The listing builds one solid part. Answer for the finished solid, in the listing's coordinates (mm). Face numbers are marked on the shaded views. A direction names the side the tool comes from. Coordinates: 2 decimals unless noted, no trailing zeros. Loops run counter-clockwise (first coordinate to the right, second up) from the corner with the lowest first, then second, coordinate; pieces in that order, holes last. Notation, with made-up numbers: (88.5, 2) - (110.5, 2) arc R12 cw to (110.5, 10) - close; hole circle Ø8 at (56.25, 55.25). An arc over 180 degrees is marked (long way). Return JSON: item names as keys, results as strings. Group by question number.
1. The mould has two halves that part along Y. Classify the marked faces 1, 2 and 3: pulls with the +Y half, pulls with the -Y half, needs draft (parallel to the pull), parting line crosses it, or undercut.
2. Which of the six approach directions +Z, -Z, +X, -X, +Y, -Y give full straight-line access (tool end or side, diameter ignored) to the marked faces 4, 5 and 6?
3. Section A-A (x = 0) is taken. Write down the section's boundary in (y, z) (3 decimals), and give its area (3 significant figures).
4. Each of these flat-tipped pins is pushed along its axis until it touches: P1, Ø11, axis at x = 2, z = 18, coming from the -Y side (3 decimals); P2, Ø4, axis at x = 3.5, y = -15.5, coming from the +Z side. Where does it stop, or does it pass through?
5. Find the intervals of material crossed by line 1 along Y through (x, z) = (0, 2) (3 decimals); line 2 along Y through (x, z) = (-5, 4) (3 decimals); line 3 along Y through (x, z) = (8.5, 15.75) (3 decimals), in increasing order.
6. Section B-B (y = -16.25) is taken. Write down the section's boundary in (x, z) (3 decimals).
7. Section C-C (z = 6) is taken. Write down the section's boundary in (x, y) (3 decimals).
8. Section D-D (y = -3) is taken. Write down the section's boundary in (x, z) (3 decimals), and give its area (3 significant figures).
```python
from build123d import *

# Parameters (mm, degrees)
F0_W      = 21.85
F0_H      = 15.85
F1_DEPTH  = 25
F3_DEPTH  = 22
F4_R      = 2.4
F5_DEPTH  = 3.001
F6_W      = 21.85
F6_H      = 14
F6_R      = 2.4
F7_DEPTH  = 3
F9_DEPTH  = 2
F11_DEPTH = 2


with BuildPart() as f1:
    # F0 (on Top) → F1 (new body)
    with BuildSketch(Plane.XY):
        Rectangle(F0_W, F0_H)
    extrude(amount=F1_DEPTH)

    # F2 (on face) → F3 (cut, through all)
    with BuildSketch(Plane.XY.offset(25)):
        with BuildLine():
            Line((3.2894660941, 3.825), (-3.2894660941, 3.825))
            ThreePointArc((-3.2894660941, 3.825), (-6.825, 3.825), (-6.825, 0.2894660941))
            Line((-6.825, 0.2894660941), (-6.825, -0.2894660941))
            ThreePointArc((-6.825, -0.2894660941), (-6.825, -3.825), (-3.2894660941, -3.825))
            Line((-3.2894660941, -3.825), (3.2894660941, -3.825))
            ThreePointArc((3.2894660941, -3.825), (6.825, -3.825), (6.825, -0.2894660941))
            Line((6.825, -0.2894660941), (6.825, 0.2894660941))
            ThreePointArc((6.825, 0.2894660941), (6.825, 3.825), (3.2894660941, 3.825))
        make_face()
    extrude(amount=-F3_DEPTH, mode=Mode.SUBTRACT)

    # F4 (on face) → F5 (cut, through all)
    with BuildSketch(Plane.XY.offset(3)):
        Circle(F4_R)
    extrude(amount=-F5_DEPTH, mode=Mode.SUBTRACT)

    # F6 (on Top) → F7 (join)
    with BuildSketch(Plane.XY):
        with Locations((0, -14.925)):
            Rectangle(F6_W, F6_H)
        with Locations((0, -14.925)):
            Circle(F6_R, mode=Mode.SUBTRACT)
    extrude(amount=F7_DEPTH)

    # F8 (on face) → F9 (join)
    with BuildSketch(Plane(origin=(-10.925, 0, 0), x_dir=(0, -1, 0), z_dir=(-1, 0, 0))):
        Polygon((21.925, 3), (7.925, 17), (7.925, 3), align=None)
    extrude(amount=-F9_DEPTH)

    # F10 (on face) → F11 (join)
    with BuildSketch(Plane.YZ.offset(10.925)):
        Polygon((-7.925, 3), (-7.925, 17), (-21.925, 3), align=None)
    extrude(amount=-F11_DEPTH)


solid = f1.part
```
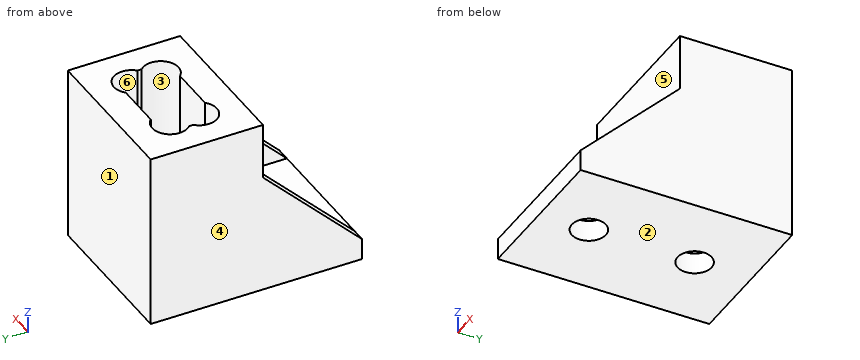
The answers:
{
 "1": {"face 1": "pulls with the +Y half", "face 2": "needs draft", "face 3": "undercut"},
 "2": {"face 4": "+Z, -Z, -X, +Y, -Y", "face 5": "+Z, -Y", "face 6": "+Z"},
 "3": {"outline": "(-21.925, 0) - (-17.325, 0) - (-17.325, 3) - (-21.925, 3) - close; (-12.525, 0) - (-2.4, 0) - (-2.4, 3) - (-3.825, 3) - (-3.825, 25) - (-7.925, 25) - (-7.925, 3) - (-12.525, 3) - close; (2.4, 0) - (7.925, 0) - (7.925, 25) - (3.825, 25) - (3.825, 3) - (2.4, 3) - close", "area": "241 mm2"},
 "4": {"P1": "stops at y = -7.925", "P2": "stops at z = 3"},
 "5": {"line 1": "y = -21.925 to -17.325, -12.525 to -2.4, 2.4 to 7.925", "line 2": "y = -7.925 to -4.557, 4.557 to 7.925", "line 3": "y = -7.925 to 7.925"},
 "6": {"outline": "(-10.925, 0) - (-2.001, 0) - (-2.001, 3) - (-8.925, 3) - (-8.925, 8.675) - (-10.925, 8.675) - close; (2.001, 0) - (10.925, 0) - (10.925, 8.675) - (8.925, 8.675) - (8.925, 3) - (2.001, 3) - close"},
 "7": {"outline": "(-10.925, -18.925) - (-8.925, -18.925) - (-8.925, -7.925) - (8.925, -7.925) - (8.925, -18.925) - (10.925, -18.925) - (10.925, 7.925) - (-10.925, 7.925) - close; hole (-6.825, -0.289) arc R2.5 ccw to (-3.289, -3.825) - (3.289, -3.825) arc R2.5 ccw to (6.825, -0.289) - (6.825, 0.289) arc R2.5 ccw to (3.289, 3.825) - (-3.289, 3.825) arc R2.5 ccw to (-6.825, 0.289) - close"},
 "8": {"outline": "(-10.925, 0) - (10.925, 0) - (10.925, 25) - (7.373, 25) - (7.373, 3) - (-7.373, 3) - (-7.373, 25) - (-10.925, 25) - close", "area": "222 mm2"}
}
